Source: CAD feature listing. Evaluate the final solid. Frame: model axes, mm. A direction names the side the tool comes from. Give positions to 0.01 mm unless a question says otherwise; leave off trailing zeros. Order: outer loops, then holes, each group sorted by start corner. A loop starts at its lowest first (then second) coordinate and runs counter-clockwise, first axis right, second up. Notation, with made-up numbers: (62.25, 43.5) - (80.25, 43.5) arc R7 cw to (80.25, 48.5) - close; hole circle Ø4 at (66, 4.25). An arc over 180 degrees is marked (long way). Use CSV: the item, a comma, the result in double quotes.
Autodesk Inventor part; units mm, degrees
ref_plane "YZ Plane" through (0, 0, 0) normal (1, 0, 0) x (0, 1, 0)
ref_plane "XZ Plane" through (0, 0, 0) normal (0, 1, 0) x (-1, 0, 0)
ref_plane "XY Plane" through (0, 0, 0) normal (0, 0, 1) x (1, 0, 0)
sketch "Skizze1" plane through (0, 0, 0) normal (1, 0, 0) x (0, 1, 0)
  line L0 (0, 0) -> (0, -15)
  line L1 (0, -15) -> (-230, -15)
  line L2 (-230, -15) -> (-230, -5)
  line L3 (-230, -5) -> (-226, -5)
  line L4 (-226, -5) -> (-226, 0)
  line L5 (-226, 0) -> (-124.5, 0)
  line L6 (-124.5, 0) -> (-124.5, -5)
  line L7 (-124.5, -5) -> (-120.5, -5)
  line L8 (-120.5, -5) -> (-120.5, 0)
  line L9 (-120.5, 0) -> (-45.5, 0)
  line L10 (-45.5, 0) -> (-45.5, -5)
  line L11 (-45.5, -5) -> (-41.5, -5)
  line L12 (-41.5, -5) -> (-41.5, 0)
  line L13 (-41.5, 0) -> (0, 0)
  dimension "d0" = 4
  dimension "d1" = 10
  dimension "d6" = 101.5
  dimension "d8" = 41.5
  dimension "d10" = 5
  dimension "d11" = 75
extrude "Extrusion1" add sketch "Skizze1" along normal blind 4
properties part number "sideHolder" material "Pappel"
Item 1: Section B-B on x = 2.75. Return the cut outline in (y, z), then the cut area to 3 significant figures.
Filled in:
outline,"(-230, -15) - (0, -15) - (0, 0) - (-41.5, 0) - (-41.5, -5) - (-45.5, -5) - (-45.5, 0) - (-120.5, 0) - (-120.5, -5) - (-124.5, -5) - (-124.5, 0) - (-226, 0) - (-226, -5) - (-230, -5) - close"
area,"3,390 mm2"
Item 2: Section A-A on z = -2.5. Return the cut outline in (x, y).
Filled in:
outline,"(0, -226) - (4, -226) - (4, -124.5) - (0, -124.5) - close; (0, -120.5) - (4, -120.5) - (4, -45.5) - (0, -45.5) - close; (0, -41.5) - (4, -41.5) - (4, 0) - (0, 0) - close"
Item 3: First-contact query: pin 1 (1 mm diameter, centred on y = -51.5, z = -7.5, fed in from -X); pin 2 (1.2 mm diameter, centred on x = 2.5, y = -122.5, fed in from +Z). Flat tips, straight axial feed; report the tip coordinate or a pass-through.
Filled in:
pin 1,"stops at x = 0"
pin 2,"stops at z = -5"
Item 4: Material intervals for line 1 (Y direction, x = 2.45, z = -0.75), sorted ascending. Write a range as from..to.
Filled in:
line 1,"y = -226..-124.5, -120.5..-45.5, -41.5..0"
Item 5: Set-up query: faces 1 (the flat face through (2, -228, -5)), 2 (the flat face through (2, -120.5, -3)), 3 (the flat face through (2, -230, -10)). Return all of +Z, -Z, +X, -X, +Y, -Y with unobstructed straight access to the full face (end or side cutting, diameter ignored); none if empty.
Filled in:
face 1,"+Z, +X, -X, -Y"
face 2,"+Z, +X, -X"
face 3,"+Z, -Z, +X, -X, -Y"
